CAD build for the part. Positions are in the model's coordinates, mm. Give positions to 0.01 mm unless a question says otherwise; leave off trailing zeros. Write each loop counter-clockwise with the first axis right and the second up, starting at its lowest first coordinate (ties: lowest second). Pieces come first, ordered by that corner, then holes. Notation, with made-up numbers: (64.5, 75) -> (102.5, 75) arc R16 cw to (102.5, 80) -> close; hole circle Ø11 at (67, -40). An arc over 180 degrees is marked (long way). Answer as a JSON object with one key per item and string values.
```python
from build123d import *

# Parameters (mm, degrees)
SKETCH2_R           = 1.5
SKETCH2_W           = 10
SKETCH2_H           = 3
BOSS_EXTRUDE1_DEPTH = 3


with BuildPart() as part:
    # Sketch2 → Boss-Extrude1 (new body)
    with BuildSketch(Plane(origin=(0, 0, 0), x_dir=(1, 0, 0), z_dir=(0, 1, 0))):
        Polygon((0, 15.5), (5, 15.5), (5, 47.5), (-45, 47.5), (-45, 15.5), (-40, 15.5), (-40, 0), (-36, 0), (-36, -3), (-26, -3), (-26, 0), (-21.5, 0), (-21.5, 3.1), (-22.8, 3.1), (-22.8, 5.6), (-21.5, 5.6), (-21.5, 9.4), (-18.5, 9.4), (-18.5, 5.6), (-17.2, 5.6), (-17.2, 3.1), (-18.5, 3.1), (-18.5, 0), (-14, 0), (-14, -3), (-4, -3), (-4, 0), (0, 0), align=None)
        with Locations(Location((-30.75, 7.9, 0), (0, 0, 270))):
            Circle(SKETCH2_R, mode=Mode.SUBTRACT)
        with Locations(Location((-9.7, 31.5, 0), (0, 0, 270))):
            Circle(SKETCH2_R, mode=Mode.SUBTRACT)
        with Locations((-9, 7.9)):
            Rectangle(SKETCH2_W, SKETCH2_H, mode=Mode.SUBTRACT)
    extrude(amount=BOSS_EXTRUDE1_DEPTH)


solid = part.part
```
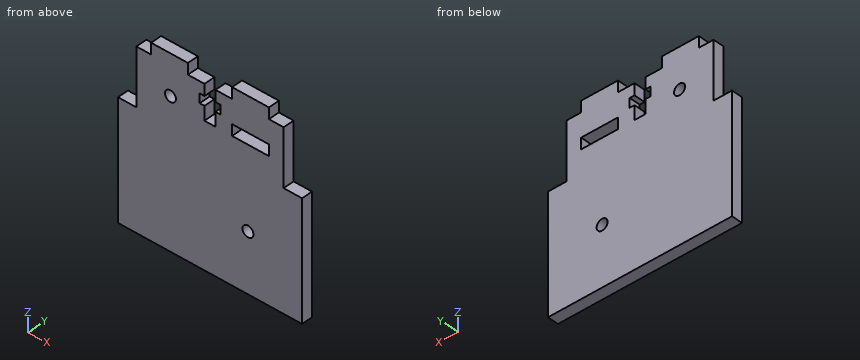
1) Slice it at A-A (x = -9.7). List the corners of the cut face in (y, z).
Model answer:
{"outline": "(0, -47.5) -> (3, -47.5) -> (3, -33) -> (0, -33) -> close; (0, -30) -> (3, -30) -> (3, -9.4) -> (0, -9.4) -> close; (0, -6.4) -> (3, -6.4) -> (3, 3) -> (0, 3) -> close"}
2) Wall check: probe 1 along X at (y, z) = (1.5, -7.9); probe 2 along X at (y, z) = (2.15, -31.5); probe 3 along Z at (x, y) = (-13.5, 1.15). Give the ranges that are in metal, low to high.
Model answer:
{"probe 1": "x = -40 to -32.25, -29.25 to -21.5, -18.5 to -14, -4 to 0", "probe 2": "x = -45 to -11.2, -8.2 to 5", "probe 3": "z = -47.5 to -9.4, -6.4 to 3"}
3) Slice it at C-C (y = 1.35). State how many separate pieces and enclosed holes the cut face has, then the cut area to 3 significant figures.
Model answer:
{"separate pieces": "1", "enclosed holes": "3", "area": "2,200 mm2"}
4) Slice it at D-D (z = -7.9). List the corners of the cut face in (x, y).
Model answer:
{"outline": "(-40, 0) -> (-32.25, 0) -> (-32.25, 3) -> (-40, 3) -> close; (-29.25, 0) -> (-21.5, 0) -> (-21.5, 3) -> (-29.25, 3) -> close; (-18.5, 0) -> (-14, 0) -> (-14, 3) -> (-18.5, 3) -> close; (-4, 0) -> (0, 0) -> (0, 3) -> (-4, 3) -> close"}
5) Slice it at B-B (z = -31.5). List the corners of the cut face in (x, y).
Model answer:
{"outline": "(-45, 0) -> (-11.2, 0) -> (-11.2, 3) -> (-45, 3) -> close; (-8.2, 0) -> (5, 0) -> (5, 3) -> (-8.2, 3) -> close"}
6) Pin check, flat tips, straight feed: pin 1 (0.9 mm diameter, centred on x = -3, y = 1.5, fed in from +Z); pin 2 (1.5 mm diameter, centred on y = 1.5, z = 1.5, fed in from +X); pin 3 (0.9 mm diameter, centred on x = 2.5, y = 1.5, fed in from +Z). Stop position of each tip, or through.
Model answer:
{"pin 1": "stops at z = 0", "pin 2": "stops at x = -4", "pin 3": "stops at z = -15.5"}
